Work out the finished part from the listing and answer in its coordinate system (mm). Round coordinates to 2 decimals unless told otherwise and drop trailing zeros. Order: outer loops, then holes, each group sorted by start corner. A loop starts at its lowest first (then second) coordinate and runs counter-clockwise, first axis right, second up. Notation, with made-up numbers: (65, 11) - (96, 11) arc R18 ccw to (96, 39) - close; hole circle Ø1 at (39.25, 59). An arc over 180 degrees is marked (long way). Use one line per item in the form item = value. Start each with the question number.
Q1. The part is cut by section B-B on z = 7.5. Determine the outline of the cut face in (x, y).
Q2. The part is cut by section A-A on x = -12.5. Determine the outline of the cut face in (y, z).
Q3. For a pull along Z with two mould halves and no side action, classify faces 1 (the flat face through (-13, 2, 222)), 2 (the cylindrical face through (-12.79, 2.03, 212.27)), 3 (the flat face through (-12, 4, 113)) as +Z half, -Z half, draft (parallel to the pull), parting line (faces both ways), or undercut.
Q4. Find the intervals of material crossed by line 1 (Z direction, x = -12.5, y = 2.6); line 2 (X direction, y = 2.4, z = 7.5), in increasing order. Write a range as [from, to].
Q5. Given P1, Ø3.5, axis at x = -12.5, z = 214.5, coming from the -Y side, flat-ended and moving along its own axis, determine where the tip first touches the part or whether it passes through.
Autodesk Inventor part; units mm, degrees
ref_plane "YZ Plane" through (0, 0, 0) normal (1, 0, 0) x (0, 1, 0)
ref_plane "XZ Plane" through (0, 0, 0) normal (0, 1, 0) x (-1, 0, 0)
ref_plane "XY Plane" through (0, 0, 0) normal (0, 0, 1) x (1, 0, 0)
sketch "Эскиз1" plane through (0, 0, 0) normal (0, 1, 0) x (-1, 0, 0)
  line L0 (0, 0) -> (25, 0)
  line L1 (25, 0) -> (25, 222)
  line L2 (25, 222) -> (0, 222)
  line L3 (0, 222) -> (0, 0)
  dimension "d0" = 25
  dimension "d1" = 222
extrude "Выдавливание1" add sketch "Эскиз1" along normal blind 4
sketch "Эскиз2" plane through (0, 4, 0) normal (0, 1, 0) x (1, 0, 0)
  circle A0 centre (-12.5, -7.5) radius 2.25
  line L0 (0, 0) -> (-25, 0)
  line L1 (0, -222) -> (0, 0)
  line L2 (0, -111) -> (-46.0375, -111)
  circle A1 centre (-12.5, -214.5) radius 2.25
  dimension "d4" = 4.5
  dimension "d5" = 7.5
extrude "Выдавливание2" cut sketch "Эскиз2" against normal blind 4
properties part number "жгут низ"
Found:
q1.outline = (-25, 0) - (-14.75, 0) - (-14.75, 4) - (-25, 4) - close; (-10.25, 0) - (0, 0) - (0, 4) - (-10.25, 4) - close
q2.outline = (0, 0) - (4, 0) - (4, 5.25) - (0, 5.25) - close; (0, 9.75) - (4, 9.75) - (4, 212.25) - (0, 212.25) - close; (0, 216.75) - (4, 216.75) - (4, 222) - (0, 222) - close
q3.face_1 = +Z half
q3.face_2 = undercut
q3.face_3 = draft
q4.line_1 = [0, 5.25], [9.75, 212.25], [216.75, 222]
q4.line_2 = [-25, -14.75], [-10.25, 0]
q5.P1 = through
